CAD build for the part. Positions are in the model's coordinates, mm. A direction names the side the tool comes from. Give positions to 0.01 mm unless a question says otherwise; leave off trailing zeros. Write each loop counter-clockwise with the first axis right and the second up, starting at its lowest first coordinate (ties: lowest second). Pieces come first, ordered by that corner, then holes. Notation, with made-up numbers: (52, -22.75) - (63, -22.75) arc R8 ccw to (63, -15.75) - close; hole circle Ø2 at (-34, 12.25). An arc over 180 degrees is marked (long way). Answer as a JSON object with one key per item and string values.
from build123d import *

# Parameters (mm, degrees)
F0_W           = 25.4
F0_H           = 9.525
F1_DEPTH       = 19.05
F2_W           = 6.35
F2_H           = 12.7
F3_DEPTH       = 25.4
F5_D           = 3.5814
F5_DEPTH       = 6.731
F5_CBORE_D     = 5.588
F5_CBORE_DEPTH = 3.175
F6_W           = 7.62
F6_H           = 12.7
F7_DEPTH       = 6.35
F8_W           = 10.16
F8_H           = 1.016
F9_DEPTH       = 12.7


with BuildPart() as f1:
    # F0 (on Top) → F1 (new body)
    with BuildSketch(Plane.XY):
        Rectangle(F0_W, F0_H)
    extrude(amount=F1_DEPTH)

    # F2 (on face) → F3 (cut)
    with BuildSketch(Plane.XZ.offset(4.7625)):
        with Locations((-9.525, 12.7)):
            Rectangle(F2_W, F2_H)
        with Locations((9.525, 12.7)):
            Rectangle(F2_W, F2_H)
    extrude(amount=-F3_DEPTH, mode=Mode.SUBTRACT)

    # F5
    with Locations(Plane.XY.offset(6.35)):
        with Locations((-9.525, 0)):
            CounterBoreHole(F5_D / 2, F5_CBORE_D / 2, F5_CBORE_DEPTH, depth=F5_DEPTH)

    # F6 (on face) → F7 (cut)
    with BuildSketch(Plane.XZ.offset(4.7625)):
        with Locations((0, 12.7)):
            Rectangle(F6_W, F6_H)
    extrude(amount=-F7_DEPTH, mode=Mode.SUBTRACT)

    # F8 (on face) → F9 (cut)
    with BuildSketch(Plane.XY.offset(19.05)):
        with Locations((0, -3.2385)):
            Rectangle(F8_W, F8_H)
    extrude(amount=-F9_DEPTH, mode=Mode.SUBTRACT)


solid = f1.part
Item 1: Probe line 1 (X direction, y = 0, z = 9.5); line 2 (X direction, y = -3.5, z = 14.5); line 3 (Y direction, x = 1.5, z = 15.75). List the from-to ranges inside material, lowest first. Write a range as from..to.
Entries:
{"line 1": "-6.35..-3.81, 3.81..6.35", "line 2": "-6.35..-5.08, 5.08..6.35", "line 3": "1.59..4.76"}
Item 2: Cut at A-A (y = 0). Give the cut face in (x, z) (3 decimals).
Entries:
{"outline": "(-12.7, 0) - (-11.316, 0) - (-11.316, 3.175) - (-12.319, 3.175) - (-12.319, 6.35) - (-12.7, 6.35) - close; (-7.734, 0) - (12.7, 0) - (12.7, 6.35) - (6.35, 6.35) - (6.35, 19.05) - (3.81, 19.05) - (3.81, 6.35) - (-3.81, 6.35) - (-3.81, 19.05) - (-6.35, 19.05) - (-6.35, 6.35) - (-6.731, 6.35) - (-6.731, 3.175) - (-7.734, 3.175) - close"}
Item 3: Flat gauge pins, fed straight in: P1, Ø5, axis at x = 8.5, y = -2, coming from the +Z side; P2, Ø3, axis at x = -9.525, y = 0, coming from the +Z side; P3, Ø1.7, axis at x = -9.5, y = -1, coming from the +Z side (3 decimals); P4, Ø4, axis at x = -0.5, z = 12, coming from the -Y side. Where does each tip first touch, or does it go through?
Entries:
{"P1": "z = 19.05", "P2": "through", "P3": "z = 3.175", "P4": "y = 1.59"}
Item 4: Cut at D-D (z = 2.25). Give the cut face in (x, y) (1 decimal).
Entries:
{"outline": "(-12.7, -4.8) - (12.7, -4.8) - (12.7, 4.8) - (-12.7, 4.8) - close; hole circle Ø3.6 at (-9.5, 0)"}
Item 5: Mould opens along Y. For faces 1 (the flat face through (-4, -3.746, 13)), 2 (the flat face through (3.81, -4, 13)), 3 (the flat face through (0, -4.762, 5)) say: +Y half, -Y half, draft (parallel to the pull), parting line (faces both ways), or undercut.
Entries:
{"face 1": "undercut", "face 2": "draft", "face 3": "-Y half"}
Item 6: Which spindle directions (+Z, -Z, +X, -X, +Y, -Y) get a long thin tool onto all of the face, cutting with end or side? Do faces 4 (the flat face through (-3.81, -1, 13)), 5 (the flat face through (9, 0, 6.35)), 6 (the flat face through (-6.35, 0, 13)), 7 (the flat face through (12.7, 0, 3)), 8 (the flat face through (-5.08, -3, 13)). Say none if no direction does.
Entries:
{"face 4": "+Z, -Y", "face 5": "+Z, +X, +Y, -Y", "face 6": "+Z, -X, +Y, -Y", "face 7": "+Z, -Z, +X, +Y, -Y", "face 8": "+Z"}
Item 7: Cut at C-C (x = -0.75). Give the cut face in (y, z), and give its area (3 significant figures).
Entries:
{"outline": "(-4.76, 0) - (4.76, 0) - (4.76, 19.05) - (1.59, 19.05) - (1.59, 6.35) - (-4.76, 6.35) - close", "area": "101 mm2"}
Item 8: Cut at B-B (z = 9.5). Give the cut face in (x, y), and give its area (3 significant figures).
Entries:
{"outline": "(-6.35, -4.76) - (-3.81, -4.76) - (-3.81, -3.75) - (-5.08, -3.75) - (-5.08, -2.73) - (-3.81, -2.73) - (-3.81, 1.59) - (3.81, 1.59) - (3.81, -2.73) - (5.08, -2.73) - (5.08, -3.75) - (3.81, -3.75) - (3.81, -4.76) - (6.35, -4.76) - (6.35, 4.76) - (-6.35, 4.76) - close", "area": "70.0 mm2"}
